from build123d import *

# Parameters (mm, degrees)
F0_R     = 44.45
F0_R_2   = 31.75
F1_DEPTH = 38.1
F2_R     = 20.184497551
F3_DEPTH = 25.4
F4_R     = 23.9709309674
F5_DEPTH = 25.654


with BuildPart() as f1:
    # F0 (on Front) → F1 (new body)
    with BuildSketch(Plane.XZ):
        Circle(F0_R)
        Circle(F0_R_2, mode=Mode.SUBTRACT)
        Circle(F0_R_2)
    extrude(amount=F1_DEPTH)

    # F2 (on face) → F3 (join)
    with BuildSketch(Plane(origin=(0, 0, 0), x_dir=(-1, 0, 0), z_dir=(0, 1, 0))):
        Circle(F2_R)
    extrude(amount=F3_DEPTH)

    # F4 (on face) → F5 (join)
    with BuildSketch(Plane.XZ.offset(38.1)):
        Circle(F4_R)
    extrude(amount=-F5_DEPTH)


solid = f1.part
The model under review builds one solid part; all positions refer to its coordinate system, in mm. A direction names the side the tool comes from. Give positions to 0.01 mm unless a question says otherwise; leave off trailing zeros. Loops run counter-clockwise (first coordinate to the right, second up) from the corner with the lowest first, then second, coordinate; pieces in that order, holes last. Notation, with made-up numbers: (1, 9.5) -> (42, 9.5) arc R27 cw to (42, 29.5) -> close; hole circle Ø5 at (53, 50.5). An arc over 180 degrees is marked (long way). Answer as a JSON object with one key per item and string values. Group by question number.
Q1. Take a section at D-D (y = 4). Write out the cut boundary in (x, z), plus the area to 3 significant figures.
Q2. Take a section at C-C (y = -21). Write out the cut boundary in (x, z).
Q3. Insertion check: pin 1 (4 mm diameter, centred on x = -14, y = -1, fed in from +Z); pin 2 (1 mm diameter, centred on x = -18, z = -11, fed in from +Y); pin 3 (12 mm diameter, centred on x = -32, y = -25, fed in from +Z). Each pin has a flat end and moves straight along its axis. Give the tip position at first contact, or say it passes through.
Q4. Take a section at A-A (z = 0). Write out the cut boundary in (x, y).
Q5. Wall thickness on line 1 along Y through (x, z) = (-40, -13); line 2 along X through (y, z) = (-13, -24.5); line 3 along X through (y, z) = (-20.5, 31.5): over which ranges is each line inside the solid? List them lowest first.
Q6. Take a section at B-B (x = 0). Write out the cut boundary in (y, z).
Q7. Tool access review of faces 1 (the cylindrical face through (4.4, 12.5, -19.7)), 2 (the flat face through (-1, -38.1, 1)): name each direction out of +Z, -Z, +X, -X, +Y, -Y from which nothing blocks a thin tool from reaching the whole face with its end or side.
Answer below:
{
 "1": {"outline": "circle Ø40.37 at (0, 0)", "area": "1,280 mm2"},
 "2": {"outline": "circle Ø88.9 at (0, 0)"},
 "3": {"pin 1": "stops at z = 42.8", "pin 2": "stops at y = 0", "pin 3": "stops at z = 36.05"},
 "4": {"outline": "(-44.45, -38.1) -> (44.45, -38.1) -> (44.45, 0) -> (20.18, 0) -> (20.18, 25.4) -> (-20.18, 25.4) -> (-20.18, 0) -> (-44.45, 0) -> close"},
 "5": {"line 1": "y = -38.1 to 0", "line 2": "x = -37.09 to 37.09", "line 3": "x = -31.36 to 31.36"},
 "6": {"outline": "(-38.1, -44.45) -> (0, -44.45) -> (0, -20.18) -> (25.4, -20.18) -> (25.4, 20.18) -> (0, 20.18) -> (0, 44.45) -> (-38.1, 44.45) -> close"},
 "7": {"face 1": "+Y", "face 2": "+Z, -Z, +X, -X, -Y"}
}
